Design review of the part built by this model. Coordinates are the model's own, in mm. A direction names the side the tool comes from. Coordinates: 2 decimals unless noted, no trailing zeros. Loops run counter-clockwise (first coordinate to the right, second up) from the corner with the lowest first, then second, coordinate; pieces in that order, holes last. Notation, with made-up numbers: (85.5, 9) - (111.5, 9) arc R28 cw to (111.5, 43) - close; hole circle Ø5 at (62.25, 67). An arc over 180 degrees is marked (long way). Answer in a Markdown table with one row per item. Add a question column.
(1) We need section D-D, the plane y = 3.9. Give the number of separate pieces and of enclosed holes in the cut face, plus the area to 3 significant figures.
(2) We need section C-C, the plane y = 22.5. Write out the cut boundary in (x, z).
(3) We need section B-B, the plane z = 1. Write out the cut boundary in (x, y).
(4) For faces 1 (the face through (11, 1, 10.95)), 2 (the face through (3.4, 25.5, 13.7)), 3 (the face through (5, 5, 11.8)), 4 (the face through (12, 30, 9.4)), 5 (the face through (8.6, 9.5, 9.3)), list the 3-axis set-ups (+Z, -Z, +X, -X, +Y, -Y) from which the entire face can be reached by the end or side of a thin tool; tool diameter is ignored.
(5) To check wall thickness, follow L1, parallel to X at y = 2.5, z = 8; L2, parallel to X at y = 8, z = 6.5; L3, parallel to X at y = 3, z = 1. State the ranges of each line that lie inside material, in increasing order. Write a range as [from, to].
(6) Clearance check with flat-ended pins moving along their axes: pin 1 (1.9 mm diameter, centred on y = 31, z = 7, fed in from -X); pin 2 (2 mm diameter, centred on x = 15, y = 7, fed in from -Z). State where each tip first meets the part, or that it passes through.
(7) We need section A-A, the plane x = 43.5. Write out the cut boundary in (y, z), plus the area to 3 significant figures.
(8) The part is to be moulded in two halves that separate along Y. For faces 6 (the face through (38.163, 2.962, 13.687)), 7 (the face through (31, 31.8, 6)), 8 (the face through (28, 27, 11.8)), say which applies: released by +Y, released by -Y, zero draft, split by the parting line, or undercut.
from build123d import *

# Parameters (mm, degrees)
F0_W      = 63.8
F0_H      = 31.8
F0_W_2    = 60.8
F0_H_2    = 28.8
F1_DEPTH  = 12.8
F2_W      = 6.3
F2_H      = 6.3
F2_W_2    = 7.8
F3_DEPTH  = 1
F4_R      = 2.45
F5_DEPTH  = 1.8
F6_W      = 0.85
F6_H      = 0.5
F7_DEPTH  = 25.4
F9_DEPTH  = 8
F11_DEPTH = 5
F12_W     = 0.1
F12_H     = 1
F13_DEPTH = 6.3
F14_W     = 6
F14_H     = 1.7
F15_DEPTH = 2.54
F16_W     = 11
F16_H     = 6
F16_W_2   = 6
F16_H_2   = 1.7
F17_DEPTH = 0.5
F19_DEPTH = 5
F21_DEPTH = 4


# Not quite as in the source:
# - a feature names something its author has since deleted; it is built from what else it names


with BuildPart() as f1:
    # F0 (on Top) → F1 (new body)
    with BuildSketch(Plane.XY):
        with Locations((31.9, 15.9)):
            Rectangle(F0_W, F0_H)
        with Locations((31.9, 15.9)):
            Rectangle(F0_W_2, F0_H_2, mode=Mode.SUBTRACT)
    extrude(amount=F1_DEPTH)

    # F2 (on face) → F3 (join)
    with BuildSketch(Plane.XY.offset(12.8)):
        with Locations((4.65, 27.15)):
            Rectangle(F2_W, F2_H)
        with Locations((4.65, 4.65)):
            Rectangle(F2_W, F2_H)
        with Locations((59.15, 4.65)):
            Rectangle(F2_W, F2_H)
        with Locations((59.15, 27.15)):
            Rectangle(F2_W, F2_H)
        with Locations((27.9, 27.15)):
            Rectangle(F2_W_2, F2_H)
        with Locations((35.9, 4.65)):
            Rectangle(F2_W_2, F2_H)
    extrude(amount=-F3_DEPTH)

    # F4 (on face) → F5 (join)
    with BuildSketch(Plane.XY.offset(12.8)):
        with Locations((3.9, 27.9)):
            Circle(F4_R)
        with Locations((59.9, 27.9)):
            Circle(F4_R)
        with Locations((59.9, 3.9)):
            Circle(F4_R)
        with Locations((3.9, 3.9)):
            Circle(F4_R)
        with Locations((27.9, 27.9)):
            Circle(F4_R)
        with Locations((35.9, 3.9)):
            Circle(F4_R)
    extrude(amount=F5_DEPTH)

    # F6 (on face) → F7 (cut)
    with BuildSketch(Plane.XZ):
        Polygon((11.575, 10.95), (9.7, 10.95), (9.7, 7.15), (14.3, 7.15), (14.3, 10.95), (12.425, 10.95), align=None)
        with Locations((12, 11.2)):
            Rectangle(F6_W, F6_H)
    extrude(amount=-F7_DEPTH, mode=Mode.SUBTRACT)

    # F8 (on face) → F9 (join)
    with BuildSketch(Plane(origin=(0, 1.5, 0), x_dir=(-1, 0, 0), z_dir=(0, 1, 0))):
        Polygon((-13.6, 5.8), (-13.6, 6.8), (-15.1, 6.8), (-15.1, 11.8), (-13.6, 11.8), (-13.6, 12.8), (-16.1, 12.8), (-16.1, 5.8), align=None)
        Polygon((-8.9, 6.8), (-10.4, 6.8), (-10.4, 5.8), (-7.9, 5.8), (-7.9, 12.8), (-10.4, 12.8), (-10.4, 11.8), (-8.9, 11.8), align=None)
    extrude(amount=F9_DEPTH)

    # F10 (on face) → F11 (join, through all)
    with BuildSketch(Plane.XY.offset(6.8)):
        Polygon((14.6, 7.6), (15.1, 7.6), (15.1, 9.5), align=None)
        Polygon((9.4, 7.6), (8.9, 9.5), (8.9, 7.6), align=None)
    extrude(amount=F11_DEPTH)

    # F12 (on face) → F13 (join, through all)
    with BuildSketch(Plane(origin=(0, 1.5, 0), x_dir=(-1, 0, 0), z_dir=(0, 1, 0))):
        with Locations((-7.85, 12.3)):
            Rectangle(F12_W, F12_H)
    extrude(amount=F13_DEPTH)

    # F14 (on face) → F15 (cut)
    with BuildSketch(Plane(origin=(0, 31.8, 0), x_dir=(-1, 0, 0), z_dir=(0, 1, 0))):
        with Locations((-12, 6.4)):
            Rectangle(F14_W, F14_H)
    extrude(amount=-F15_DEPTH, mode=Mode.SUBTRACT)

    # F16 (on face) → F17 (join)
    with BuildSketch(Plane.XZ.offset(-30.3)):
        with Locations((12, 6.4)):
            Rectangle(F16_W, F16_H)
        with Locations((12, 6.4)):
            Rectangle(F16_W_2, F16_H_2, mode=Mode.SUBTRACT)
    extrude(amount=F17_DEPTH)

    # F18 (on face) → F19 (join)
    with BuildSketch(Plane.XZ.offset(-29.8)):
        Polygon((9, 9.4), (6.5, 9.4), (6.5, 3.4), (9, 3.4), (9, 4.4), (7.5, 4.4), (7.5, 8.4), (9, 8.4), align=None)
        Polygon((17.5, 9.4), (15, 9.4), (15, 8.4), (16.5, 8.4), (16.5, 4.4), (15, 4.4), (15, 3.4), (17.5, 3.4), align=None)
    extrude(amount=F19_DEPTH)

    # F20 (on face) → F21 (join, through all)
    with BuildSketch(Plane.XY.offset(4.4)):
        Polygon((7.5, 25.8), (7.5, 24.8), (8, 25.8), align=None)
        Polygon((16, 25.8), (16.5, 24.8), (16.5, 25.8), align=None)
    extrude(amount=F21_DEPTH)


solid = f1.part
Responses:
| question | item | result |
|---|---|---|
| 1 | separate pieces | 4 |
| 1 | enclosed holes | 0 |
| 1 | area | 105 mm2 |
| 2 | outline | (0, 0) - (1.5, 0) - (1.5, 12.8) - (0, 12.8) - close; (62.3, 0) - (63.8, 0) - (63.8, 12.8) - (62.3, 12.8) - close |
| 3 | outline | (0, 0) - (63.8, 0) - (63.8, 31.8) - (0, 31.8) - close; hole (1.5, 1.5) - (62.3, 1.5) - (62.3, 30.3) - (1.5, 30.3) - close |
| 4 | face 1 | -Y |
| 4 | face 2 | +Z |
| 4 | face 3 | -Z |
| 4 | face 4 | none |
| 4 | face 5 | +Z, -Z |
| 5 | L1 | x = [0, 1.5], [7.9, 8.9], [15.1, 16.1], [62.3, 63.8] |
| 5 | L2 | x = [0, 1.5], [7.9, 10.4], [13.6, 16.1], [62.3, 63.8] |
| 5 | L3 | x = [0, 1.5], [62.3, 63.8] |
| 6 | pin 1 | stops at x = 0 |
| 6 | pin 2 | stops at z = 5.8 |
| 7 | outline | (0, 0) - (1.5, 0) - (1.5, 12.8) - (0, 12.8) - close; (30.3, 0) - (31.8, 0) - (31.8, 12.8) - (30.3, 12.8) - close |
| 7 | area | 38.4 mm2 |
| 8 | face 6 | split by the parting line |
| 8 | face 7 | released by +Y |
| 8 | face 8 | undercut |
